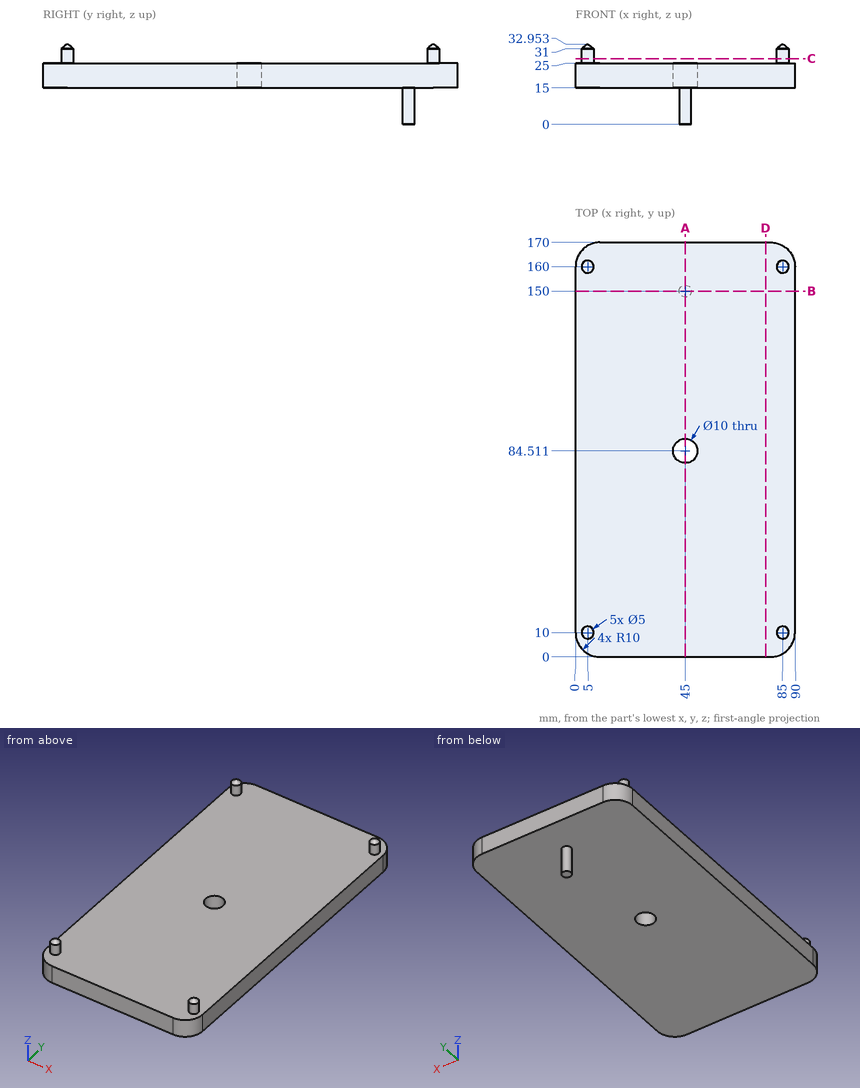
The drawing under review shows one solid part. Ordinate dimensions are in mm from its lowest x, y, z. Round coordinates to 2 decimals unless told otherwise and drop trailing zeros. Loops run counter-clockwise (first coordinate to the right, second up) from the corner with the lowest first, then second, coordinate; pieces in that order, holes last. Notation, with made-up numbers: (-20, -35) -> (-11, -35) arc R17 ccw to (-11, -14) -> close; hole circle Ø4 at (-5.5, -6). An arc over 180 degrees is marked (long way). One line per question, with ' | ' between items. Start each with the question number.
Item 1: Wall thickness on line 1 along Y through (x, z) = (45, 21); line 2 along Z through (x, y) = (23.5, 134); line 3 along X through (y, z) = (83.5, 20.5): over which ranges is each line inside the solid? List them lowest first. Write a range as [from, to].
Item 2: Add section A-A, the plane x = 45. Write out the cut boundary in (y, z), then the cut area to 4 significant figures.
Item 3: Add section C-C, the plane z = 27. Write out the cut boundary in (x, y).
Item 4: Add section B-B, the plane y = 150. Write out the cut boundary in (x, z), then the cut area to 3 significant figures.
Item 5: For pin 1 (6 mm diameter, centred on x = 74, z = 13, fed in from +Y); pin 2 (8 mm diameter, centred on x = 35.5, y = 114.5, fed in from -Z); pin 3 (6 mm diameter, centred on x = 45, y = 84.51, fed in from -Z), all flat-tipped, find the tip position at first contact; note any pin that passes through.
Item 6: Add section D-D, the plane x = 78. Write out the cut boundary in (y, z), then the cut area to 3 significant figures.
Return value:
1) line 1: y = [0, 79.51], [89.51, 170] | line 2: z = [15, 25] | line 3: x = [0, 40.1], [49.9, 90]
2) outline: (0, 15) -> (79.51, 15) -> (79.51, 25) -> (0, 25) -> close; (89.51, 15) -> (147.5, 15) -> (147.5, 0) -> (152.5, 0) -> (152.5, 15) -> (170, 15) -> (170, 25) -> (89.51, 25) -> close | area: 1,675 mm2
3) outline: circle Ø5 at (5, 10); circle Ø5 at (5, 160); circle Ø5 at (85, 10); circle Ø5 at (85, 160)
4) outline: (0, 15) -> (42.5, 15) -> (42.5, 0) -> (47.5, 0) -> (47.5, 15) -> (90, 15) -> (90, 25) -> (0, 25) -> close | area: 975 mm2
5) pin 1: stops at y = 170 | pin 2: stops at z = 15 | pin 3: passes through
6) outline: (0, 15) -> (170, 15) -> (170, 25) -> (0, 25) -> close | area: 1,700 mm2
